```python
from build123d import *

# Parameters (mm, degrees)
F0_W        = 168.1647002697
F0_H        = 22.3620980978
F1_DEPTH    = 25.4
F2_W        = 86.963314563
F2_H        = 11.1810490489
F3_DEPTH    = 25.4
F4_T1_DEPTH = 25.4
F5_T1_DEPTH = 25.4
F6_R        = 2.54


# Not quite as in the source:
# - a fillet or chamfer that OpenCascade refuses, or shapes differently, is made with other operations: its cross-section is extruded or revolved along the edge and cut away or added


with BuildPart() as f1:
    # F0 (on Front) → F1 (new body)
    with BuildSketch(Plane.XZ):
        Rectangle(F0_W, F0_H)
    extrude(amount=F1_DEPTH)

    # F2 (on face) → F3 (cut)
    with BuildSketch(Plane.XZ.offset(25.4)):
        with Locations((0.4539322108, -5.5905245245)):
            Rectangle(F2_W, F2_H)
    extrude(amount=-F3_DEPTH, mode=Mode.SUBTRACT)

    # F4: fillet of radius 12.7 on 1 edges, made by hand

    # F4_s2 → F4_t1 (join)
    with BuildSketch(Plane.XZ):
        with BuildLine():
            ThreePointArc((-43.0277250707, -11.1810490489), (-38.8450170607, -3.1978771562), (-30.4188873761, 0))
            Line((-30.4188873761, 0), (-43.0277250707, 0))
            Line((-43.0277250707, 0), (-43.0277250707, -11.1810490489))
        make_face()
    extrude(amount=F4_T1_DEPTH)

    # F5: fillet of radius 12.7 on 1 edges, made by hand

    # F5_s2 → F5_t1 (join)
    with BuildSketch(Plane.XZ):
        with BuildLine():
            ThreePointArc((43.9355894923, -11.1810490489), (39.7528814823, -3.1978771562), (31.3267517977, 0))
            Line((31.3267517977, 0), (43.9355894923, 0))
            Line((43.9355894923, 0), (43.9355894923, -11.1810490489))
        make_face()
    extrude(amount=F5_T1_DEPTH)

    # F6
    f6_edges = [f1.edges().sort_by_distance(p)[0] for p in [
        (0, -25.4, 11.181049),
    ]]
    fillet(f6_edges, radius=F6_R)


solid = f1.part
```
Here's how the part is built. I have some questions about the finished solid (model axes, mm). A direction names the side the tool comes from. Round coordinates to 2 decimals unless told otherwise and drop trailing zeros. Write each loop counter-clockwise with the first axis right and the second up, starting at its lowest first coordinate (ties: lowest second). Pieces come first, ordered by that corner, then holes.
Q1. Please list where these lines run through material, in increasing order: probe 1 along Z at (x, y) = (8, -2.5); probe 2 along Z at (x, y) = (-55.5, -23); probe 3 along X at (y, z) = (-14.75, -2.5).
Q2. If we mould it in two halves opening along X, with no side actions, what happens to faces 3 (the cylindrical face through (39.849, -12.522, -3.284)), 4 (the flat face through (-84.082, -13, 0)), 5 (the flat face through (-1, -11, 11.181)), 6 (the cylindrical face through (-38.941, -12.522, -3.284))? For each: +X half, -X half, draft (parallel to the pull), parting line (faces both ways), or undercut.
Q3. Will this pin go through, and if not, where does the flat tip stop? P1, Ø5, axis at x = 7.5, y = -8.5, coming from the -Z side.
Q4. If we section it at D-D on z = -3: Write out the boundary of the cut face in (x, y), plus the area to 3 significant figures.
Q5. Which directions (+Z, -Z, +X, -X, +Y, -Y) give clear straight access to the entire face, cutting with the end or side of a thin tool? Please do faces 1 (the flat face through (0, -13, 0)), 2 (the flat face through (84.082, -13, 0)).
Q6. If we section it at B-B on x = 10: Write out the boundary of the cut face in (y, z), plus the area to 3 significant figures.
Q7. If we section it at A-A on z = -9.25: Write out the boundary of the cut face in (x, y).
Q8. If we section it at C-C on y = -11.25: Write out the boundary of the cut face in (x, z).
Answer below:
1. probe 1: z = 0 to 11.18
1. probe 2: z = -11.18 to 11.18
1. probe 3: x = -84.08 to -37.99, 38.89 to 84.08
2. face 3: undercut
2. face 4: -X half
2. face 5: draft
2. face 6: undercut
3. P1: stops at z = 0
4. outline: (-84.08, -25.4) - (-38.62, -25.4) - (-38.62, 0) - (-84.08, 0) - close; (39.52, -25.4) - (84.08, -25.4) - (84.08, 0) - (39.52, 0) - close
4. area: 2,290 mm2
5. face 1: -Z, +Y, -Y
5. face 2: +Z, -Z, +X, +Y, -Y
6. outline: (-25.4, 0) - (0, 0) - (0, 11.18) - (-22.86, 11.18) arc R2.54 ccw to (-25.4, 8.64) - close
6. area: 283 mm2
7. outline: (-84.08, -25.4) - (-42.64, -25.4) - (-42.64, 0) - (-84.08, 0) - close; (43.55, -25.4) - (84.08, -25.4) - (84.08, 0) - (43.55, 0) - close
8. outline: (-84.08, -11.18) - (-43.03, -11.18) arc R12.7 cw to (-30.42, 0) - (31.33, 0) arc R12.7 cw to (43.94, -11.18) - (84.08, -11.18) - (84.08, 11.18) - (-84.08, 11.18) - close
